```python
from build123d import *

# Parameters (mm, degrees)
BOSS_EXTRUDE1_DEPTH = 10.11
SKETCH1_3_R         = 4
BOSS_EXTRUDE2_DEPTH = 2
CUT_EXTRUDE1_REACH  = 22
SKETCH3_R           = 3


with BuildPart() as part:
    # Sketch1 → Boss-Extrude1 (new body)
    with BuildSketch(Plane.XZ.offset(5.655564884)):
        with BuildLine():
            Line((-3.830791813, -12.996740626), (-3.830791813, 1.003259374))
            ThreePointArc((-3.830791813, 1.003259374), (-5.002364688, 3.831686499), (-7.830791813, 5.003259374))
            Line((-7.830791813, 5.003259374), (-19.830791813, 5.003259374))
            ThreePointArc((-19.830791813, 5.003259374), (-22.659218938, 3.831686499), (-23.830791813, 1.003259374))
            Line((-23.830791813, 1.003259374), (-23.830791813, -12.996740626))
            ThreePointArc((-23.830791813, -12.996740626), (-22.659218938, -15.825167751), (-19.830791813, -16.996740626))
            Line((-19.830791813, -16.996740626), (-7.830791813, -16.996740626))
            ThreePointArc((-7.830791813, -16.996740626), (-5.002364688, -15.825167751), (-3.830791813, -12.996740626))
        make_face()
        with BuildLine():
            ThreePointArc((-21.830791813, -12.996740626), (-21.245005376, -14.410954188), (-19.830791813, -14.996740626))
            Line((-19.830791813, -14.996740626), (-7.830791813, -14.996740626))
            ThreePointArc((-7.830791813, -14.996740626), (-6.416578251, -14.410954188), (-5.830791813, -12.996740626))
            Line((-5.830791813, -12.996740626), (-5.830791813, 1.003259374))
            ThreePointArc((-5.830791813, 1.003259374), (-6.416578251, 2.417472937), (-7.830791813, 3.003259374))
            Line((-7.830791813, 3.003259374), (-19.830791813, 3.003259374))
            ThreePointArc((-19.830791813, 3.003259374), (-21.245005376, 2.417472937), (-21.830791813, 1.003259374))
            Line((-21.830791813, 1.003259374), (-21.830791813, -12.996740626))
        make_face(mode=Mode.SUBTRACT)
    extrude(amount=-BOSS_EXTRUDE1_DEPTH)

    # Sketch1_3 → Boss-Extrude2 (add)
    with BuildSketch(Plane.XZ.offset(5.655564884)):
        with BuildLine():
            Line((-7.830791813, 5.003259374), (-19.830791813, 5.003259374))
            ThreePointArc((-19.830791813, 5.003259374), (-22.659218938, 3.831686499), (-23.830791813, 1.003259374))
            Line((-23.830791813, 1.003259374), (-23.830791813, -12.996740626))
            ThreePointArc((-23.830791813, -12.996740626), (-22.659218938, -15.825167751), (-19.830791813, -16.996740626))
            Line((-19.830791813, -16.996740626), (-7.830791813, -16.996740626))
            ThreePointArc((-7.830791813, -16.996740626), (-5.002364688, -15.825167751), (-3.830791813, -12.996740626))
            Line((-3.830791813, -12.996740626), (-3.830791813, 1.003259374))
            ThreePointArc((-3.830791813, 1.003259374), (-5.002364688, 3.831686499), (-7.830791813, 5.003259374))
        make_face()
        with Locations((-13.830791813, -1.996740626)):
            Circle(SKETCH1_3_R, mode=Mode.SUBTRACT)
    extrude(amount=BOSS_EXTRUDE2_DEPTH)

    # Sketch3 → Cut-Extrude1 (cut, up to next)
    with BuildSketch(Plane.ZY.offset(3.830791813), mode=Mode.PRIVATE) as cut_extrude1_sk1:
        with Locations((-9.996740626, -0.545564884)):
            Circle(SKETCH3_R)
    cut_extrude1_tool1 = extrude(cut_extrude1_sk1.sketch, amount=CUT_EXTRUDE1_REACH, mode=Mode.PRIVATE) & part.part
    add(cut_extrude1_tool1.solids().sort_by_distance((-3.830792, -0.545565, -9.996741))[0], mode=Mode.SUBTRACT)


solid = part.part
```
Design review of the part built by this model. Coordinates are the model's own, in mm. A direction names the side the tool comes from. Coordinates: 2 decimals unless noted, no trailing zeros. Order: outer loops, then holes, each group sorted by start corner. A loop starts at its lowest first (then second) coordinate and runs counter-clockwise, first axis right, second up. Notation, with made-up numbers: M 56.25,80.5 L 96.25,80.5 A32 ccw 96.25,118.5 Z; hole C 49.25,-14.5 d5. An arc over 180 degrees is marked long. Answer as a JSON object with one key per item and string values. Group by question number.
1) Add section C-C, the plane x = -19.5. Write out the cut boundary in (y, z), then the cut area to 3 significant figures.
2) Add section A-A, the plane y = 3.5. Write out the cut boundary in (x, z), then the cut area to 3 significant figures.
3) Tool access review of faces 4 (the flat face through (-5.831, -1, -5)), 5 (the cylindrical face through (-4.97, -1.52, 3.8)): name each direction out of +Z, -Z, +X, -X, +Y, -Y from which nothing blocks a thin tool from reaching the whole face with its end or side.
4) For pin 1 (5 mm diameter, centred on x = -13, z = -9.5, fed in from +Y); pin 2 (3 mm diameter, centred on y = -3, z = -9, fed in from +X), all flat-tipped, find the tip position at first contact; note any pin that passes through.
5) Add section D-D, the plane z = -11.25. Write out the cut boundary in (x, y), then the cut area to 3 significant figures.
6) Wall thickness on L1, parallel to Z at x = -9.25, y = -4; L2, parallel to X at y = 0.25, z = -2; L3, parallel to Y at x = -12.25, z = -14.75: over which ranges is each line inside the solid? List them lowest first.
7) Add section B-B, the plane x = -15.5. Write out the cut boundary in (y, z).
8) Mouldability with a two-part tool opening along Y and no side actions: class faces 1 (the cylindrical face through (-4.817, 0.356, -7.135)), 2 (the cylindrical face through (-11.99, -6.64, -5.55)), 3 (the flat face through (-14, -5.656, -8)) as pulls with the +Y half, pulls with the -Y half, needs draft (parallel to the pull), parting line crosses it, or undercut.
Computed values:
{
 "1": {"outline": "M -7.66,-17 L 4.45,-17 L 4.45,-15 L -5.66,-15 L -5.66,3 L 4.45,3 L 4.45,5 L -7.66,5 Z", "area": "84.4 mm^2"},
 "2": {"outline": "M -23.83,-13 A4 ccw -19.83,-17 L -7.83,-17 A4 ccw -3.83,-13 L -3.83,1 A4 ccw -7.83,5 L -19.83,5 A4 ccw -23.83,1 Z; hole M -21.83,-13 A2 ccw -19.83,-15 L -7.83,-15 A2 ccw -5.83,-13 L -5.83,1 A2 ccw -7.83,3 L -19.83,3 A2 ccw -21.83,1 Z", "area": "142 mm^2"},
 "3": {"face 4": "+Y", "face 5": "+Z, +X, +Y, -Y"},
 "4": {"pin 1": "stops at y = -5.66", "pin 2": "stops at x = -3.83"},
 "5": {"outline": "M -23.83,-7.66 L -3.83,-7.66 L -3.83,-3.27 L -5.83,-3.27 L -5.83,-5.66 L -21.83,-5.66 L -21.83,4.45 L -23.83,4.45 Z; M -5.83,2.18 L -3.83,2.18 L -3.83,4.45 L -5.83,4.45 Z", "area": "69.5 mm^2"},
 "6": {"L1": "z = -17 to -15, 3 to 5", "L2": "x = -23.83 to -21.83, -5.83 to -3.83", "L3": "y = -7.66 to -5.66"},
 "7": {"outline": "M -7.66,-17 L 4.45,-17 L 4.45,-15 L -5.66,-15 L -5.66,-5.63 L -7.66,-5.63 Z; M -7.66,1.64 L -5.66,1.64 L -5.66,3 L 4.45,3 L 4.45,5 L -7.66,5 Z"},
 "8": {"face 1": "undercut", "face 2": "needs draft", "face 3": "pulls with the +Y half"}
}
